Check sheet for the modelled part. Datum: model origin and axes. Units: mm. Round coordinates to 2 decimals unless told otherwise and drop trailing zeros. One line per item, written item: value.
from build123d import *

# Parameters (mm, degrees)
SKETCH_1_W             = 129
SKETCH_1_H             = 86
EXTRUDE_2_DEPTH        = 2.73
CUT_EXTRUDE_1507_DEPTH = 1
SKETCH_1_7_RX          = 0.202164981
SKETCH_1_7_RY          = 0.2
CUT_EXTRUDE_5_DEPTH    = 0.3
CUT_EXTRUDE_15_DEPTH   = 0.3


with BuildPart() as part:
    # Sketch 1 → Extrude 2 (new body)
    with BuildSketch(Plane(origin=(0, 0, 0), x_dir=(1, 0, 0), z_dir=(0, 1, 0))):
        with Locations((62.5, 41)):
            Rectangle(SKETCH_1_W, SKETCH_1_H)
    extrude(amount=EXTRUDE_2_DEPTH)

    # Sketch 1_4 → Cut-Extrude 1507 (cut)
    with BuildSketch(Plane(origin=(0, 0, 0), x_dir=(1, 0, 0), z_dir=(0, 1, 0))):
        with BuildLine():
            Line((6.5, -1.607315502), (6.5, 77.9))
            ThreePointArc((6.5, 77.9), (6.646446609, 78.253553391), (7, 78.4))
            Line((7, 78.4), (25, 78.4))
            ThreePointArc((25, 78.4), (25.353553391, 78.253553391), (25.5, 77.9))
            Line((25.5, 77.9), (25.5, 3.9))
            ThreePointArc((25.5, 3.9), (25.646446609, 3.546446609), (26, 3.4))
            Line((26, 3.4), (42, 3.4))
            ThreePointArc((42, 3.4), (42.353553391, 3.546446609), (42.5, 3.9))
            Line((42.5, 3.9), (42.5, 77.9))
            ThreePointArc((42.5, 77.9), (42.646446609, 78.253553391), (43, 78.4))
            Line((43, 78.4), (61, 78.4))
            ThreePointArc((61, 78.4), (61.353553391, 78.253553391), (61.5, 77.9))
            Line((61.5, 77.9), (61.5, 3.9))
            ThreePointArc((61.5, 3.9), (61.646446609, 3.546446609), (62, 3.4))
            Line((62, 3.4), (78, 3.4))
            ThreePointArc((78, 3.4), (78.353553391, 3.546446609), (78.5, 3.9))
            Line((78.5, 3.9), (78.5, 77.9))
            ThreePointArc((78.5, 77.9), (78.646446609, 78.253553391), (79, 78.4))
            Line((79, 78.4), (97, 78.4))
            ThreePointArc((97, 78.4), (97.353553391, 78.253553391), (97.5, 77.9))
            Line((97.5, 77.9), (97.5, 3.9))
            ThreePointArc((97.5, 3.9), (97.646446609, 3.546446609), (98, 3.4))
            Line((98, 3.4), (114, 3.4))
            ThreePointArc((114, 3.4), (114.353553391, 3.546446609), (114.5, 3.9))
            Line((114.5, 3.9), (114.5, 78.4))
            Line((114.5, 78.4), (114.5, 83))
            Line((114.5, 83), (115.5, 83))
            Line((115.5, 83), (115.5, 77.4))
            Line((115.5, 77.4), (115.5, 2.9))
            ThreePointArc((115.5, 2.9), (115.353553391, 2.546446609), (115, 2.4))
            Line((115, 2.4), (97, 2.4))
            ThreePointArc((97, 2.4), (96.646446609, 2.546446609), (96.5, 2.9))
            Line((96.5, 2.9), (96.5, 76.9))
            ThreePointArc((96.5, 76.9), (96.353553391, 77.253553391), (96, 77.4))
            Line((96, 77.4), (80, 77.4))
            ThreePointArc((80, 77.4), (79.646446609, 77.253553391), (79.5, 76.9))
            Line((79.5, 76.9), (79.5, 2.9))
            ThreePointArc((79.5, 2.9), (79.353553391, 2.546446609), (79, 2.4))
            Line((79, 2.4), (61, 2.4))
            ThreePointArc((61, 2.4), (60.646446609, 2.546446609), (60.5, 2.9))
            Line((60.5, 2.9), (60.5, 76.9))
            ThreePointArc((60.5, 76.9), (60.353553391, 77.253553391), (60, 77.4))
            Line((60, 77.4), (44, 77.4))
            ThreePointArc((44, 77.4), (43.646446609, 77.253553391), (43.5, 76.9))
            Line((43.5, 76.9), (43.5, 2.9))
            ThreePointArc((43.5, 2.9), (43.353553391, 2.546446609), (43, 2.4))
            Line((43, 2.4), (25, 2.4))
            ThreePointArc((25, 2.4), (24.646446609, 2.546446609), (24.5, 2.9))
            Line((24.5, 2.9), (24.5, 76.9))
            ThreePointArc((24.5, 76.9), (24.353553391, 77.253553391), (24, 77.4))
            Line((24, 77.4), (8, 77.4))
            ThreePointArc((8, 77.4), (7.646446609, 77.253553391), (7.5, 76.9))
            Line((7.5, 76.9), (7.5, -1.607315502))
            Line((7.5, -1.607315502), (6.5, -1.607315502))
        make_face()
    extrude(amount=CUT_EXTRUDE_1507_DEPTH, mode=Mode.SUBTRACT)

    # Sketch 1_7 → Cut-Extrude 5 (cut)
    with BuildSketch(Plane(origin=(0, 0, 0), x_dir=(1, 0, 0), z_dir=(0, 1, 0))):
        with Locations(Location((16, 41), (0, 0, 180))):
            Ellipse(SKETCH_1_7_RX, SKETCH_1_7_RY)
    extrude(amount=CUT_EXTRUDE_5_DEPTH, mode=Mode.SUBTRACT)

    # Sketch 9 → Cut-Extrude 15 (cut)
    with BuildSketch(Plane(origin=(0, 0, 0), x_dir=(1, 0, 0), z_dir=(0, 1, 0))):
        with BuildLine():
            Line((15.847835019, 40.868322065), (15.847835019, -2))
            Line((15.847835019, -2), (16.152164981, -2))
            Line((16.152164981, -2), (16.152164981, 40.868322065))
            add(Edge.make_bspline(
                [(15.847835019, 40.868322065), (16, 40.696228529), (16.152164981, 40.868322065)],
                knots=[0.71867729, 0.71867729, 0.71867729, 2.422915364, 2.422915364, 2.422915364], degree=2, weights=[1, 0.658389675, 1]))
        make_face()
        with BuildLine():
            add(Edge.make_bspline(
                [(51.847835019, 40.868322065), (52, 40.696228529), (52.152164981, 40.868322065)],
                knots=[0.71867729, 0.71867729, 0.71867729, 2.422915364, 2.422915364, 2.422915364], degree=2, weights=[1, 0.658389675, 1]))
            Line((51.847835019, 40.868322065), (51.847835019, -2))
            Line((51.847835019, -2), (52.152164981, -2))
            Line((52.152164981, -2), (52.152164981, 40.868322065))
        make_face()
        with BuildLine():
            Line((70.664301479, 83), (70.364301479, 83))
            Line((70.364301479, 83), (70.335776261, 41.114151494))
            ThreePointArc((70.335776261, 41.114151494), (70.500068136, 41.199999988), (70.664301479, 41.114039572))
            Line((70.664301479, 41.114039572), (70.664301479, 83))
        make_face()
        with BuildLine():
            ThreePointArc((70.664301479, 41.114039572), (70.500068136, 41.199999988), (70.335776261, 41.114151494))
            Line((70.335776261, 41.114151494), (70.335698521, 41))
            Line((70.335698521, 41), (70.664301479, 41))
            Line((70.664301479, 41), (70.664301479, 41.114039572))
        make_face()
        with BuildLine():
            Line((70.335698521, 41), (70.335776261, 41.114151494))
            ThreePointArc((70.335776261, 41.114151494), (70.44018674, 40.809153533), (70.7, 41))
            ThreePointArc((70.7, 41), (70.690866833, 41.059748239), (70.664301479, 41.114039572))
            Line((70.664301479, 41.114039572), (70.664301479, 41))
            Line((70.664301479, 41), (70.335698521, 41))
        make_face()
        with BuildLine():
            Line((51.847835019, 40.868322065), (51.847835019, 41))
            Line((51.847835019, 41), (52.152164981, 41))
            Line((52.152164981, 41), (52.152164981, 40.868322065))
            add(Edge.make_bspline(
                [(52.152164981, 40.868322065), (52.344349714, 41.085676609), (52.071092366, 41.187225919), (51.797835019, 41.288775229), (51.797835019, 41)],
                knots=[2.422915364, 2.422915364, 2.422915364, 4.353050335, 4.353050335, 6.283185307, 6.283185307, 6.283185307], degree=2, weights=[1, 0.569361398, 1, 0.569361398, 1]))
            add(Edge.make_bspline(
                [(51.797835019, 41), (51.797835019, 40.924870403), (51.847835019, 40.868322065)],
                knots=[0, 0, 0, 0.71867729, 0.71867729, 0.71867729], degree=2, weights=[1, 0.936129597, 1]))
        make_face()
        with BuildLine():
            Line((52.152164981, 41), (51.847835019, 41))
            Line((51.847835019, 41), (51.847835019, 40.868322065))
            add(Edge.make_bspline(
                [(51.847835019, 40.868322065), (52, 40.696228529), (52.152164981, 40.868322065)],
                knots=[0.71867729, 0.71867729, 0.71867729, 2.422915364, 2.422915364, 2.422915364], degree=2, weights=[1, 0.658389675, 1]))
            Line((52.152164981, 40.868322065), (52.152164981, 41))
        make_face()
        with BuildLine():
            add(Edge.make_bspline(
                [(15.797835019, 41), (15.797835019, 40.924870403), (15.847835019, 40.868322065)],
                knots=[0, 0, 0, 0.71867729, 0.71867729, 0.71867729], degree=2, weights=[1, 0.936129597, 1]))
            Line((15.847835019, 40.868322065), (15.847835019, 41))
            Line((15.847835019, 41), (16.152164981, 41))
            Line((16.152164981, 41), (16.152164981, 40.868322065))
            add(Edge.make_bspline(
                [(16.152164981, 40.868322065), (16.344349714, 41.085676609), (16.071092366, 41.187225919), (15.797835019, 41.288775229), (15.797835019, 41)],
                knots=[2.422915364, 2.422915364, 2.422915364, 4.353050335, 4.353050335, 6.283185307, 6.283185307, 6.283185307], degree=2, weights=[1, 0.569361398, 1, 0.569361398, 1]))
        make_face()
        with BuildLine():
            Line((15.847835019, 41), (15.847835019, 40.868322065))
            add(Edge.make_bspline(
                [(15.847835019, 40.868322065), (16, 40.696228529), (16.152164981, 40.868322065)],
                knots=[0.71867729, 0.71867729, 0.71867729, 2.422915364, 2.422915364, 2.422915364], degree=2, weights=[1, 0.658389675, 1]))
            Line((16.152164981, 40.868322065), (16.152164981, 41))
            Line((16.152164981, 41), (15.847835019, 41))
        make_face()
    extrude(amount=CUT_EXTRUDE_15_DEPTH, mode=Mode.SUBTRACT)


solid = part.part
Item 1: Depth check by flat-ended pin: P1, Ø2, axis at x = 11.5, z = -19.5, coming from the -Y side. Enter the tip coordinate at first touch or a pass-through.
Answer:
P1: stops at y = 0
Item 2: Thickness scan on line 1 (X direction, y = 0.2, z = -2); line 2 (Z direction, x = 70.5, y = 0.15); line 3 (Z direction, x = 16.5, y = 0.4). Record the ranges inside material, lowest first.
Answer:
line 1: x = -2 to 6.5, 7.5 to 15.85, 16.15 to 51.85, 52.15 to 127
line 2: z = -84 to -83, -40.8 to -3.4, -2.4 to 2
line 3: z = -84 to -78.4, -77.4 to 2
Item 3: Mould release check, pull along Z, two halves, no side actions. Record for faces 1 (the flat face through (62, 1, -84)), 2 (the flat face through (62, 0, -42)), 3 (the flat face through (62, 1, 2)), 4 (the flat face through (61, 1, -31)): pulls with the +Z half, pulls with the -Z half, needs draft (parallel to the pull), parting line crosses it, or undercut.
Answer:
face 1: pulls with the -Z half
face 2: needs draft
face 3: pulls with the +Z half
face 4: undercut
